Could you check a few things on this model? Use its own coordinates, in mm. Round coordinates to 2 decimals unless told otherwise and drop trailing zeros. Loops run counter-clockwise (first coordinate to the right, second up) from the corner with the lowest first, then second, coordinate; pieces in that order, holes last. Notation, with made-up numbers: M 50,17.5 L 70,17.5 A22 ccw 70,27.5 Z; hole C 82,-33 d4. An arc over 180 degrees is marked long. Return JSON: item names as keys, results as strings. Group by question number.
Autodesk Inventor part; units mm, degrees
ref_plane "Начальная плоскость" through (0, 0, -68.5714) normal (0, 0, 1) x (1, 0, 0)
ref_plane "Конечная плоскость" through (0, 0, 2801.8221) normal (0, 0, 1) x (1, 0, 0)
ref_plane "РабПлоскость4" through (91.07, -73.4212, 2735.6598) normal (0, -0.5039, 0.8638) x (1, 0, 0)
ref_plane "Начальная плоскость" through (0, 0, -68.5714) normal (0, 0, 1) x (1, 0, 0)
ref_plane "Конечная плоскость" through (0, 0, 2801.8221) normal (0, 0, 1) x (1, 0, 0)
sketch "Эскиз" plane through (0, 0, 0) normal (0, 0, 1) x (1, 0, 0)
  line L0 (-1.43, 0) -> (-1.43, 40)
  line L1 (-1.43, 40) -> (43.57, 40)
  line L2 (43.57, 40) -> (43.57, 38.1774)
  line L3 (39.9881, 34.1993) -> (11.2338, 31.1771)
  line L4 (4.07, 23.221) -> (4.07, 0)
  line L5 (4.07, 0) -> (-1.43, 0) construction
  line L6 (23.82, 40) -> (23.82, 32.5) construction
  line L7 (43.57, 34.5758) -> (43.57, 32.5) construction
  line L8 (43.57, 32.5) -> (23.82, 32.5) construction
  line L9 (0, 15) -> (0, -27) construction
  line L10 (-5.539, 0) -> (16.0067, 0) construction
  line L11 (-1.43, 0) -> (-1.43, -40)
  line L12 (-1.43, -40) -> (43.57, -40)
  line L13 (43.57, -40) -> (43.57, -38.1774)
  line L14 (39.9881, -34.1993) -> (11.2338, -31.1771)
  line L15 (4.07, -23.221) -> (4.07, 0)
  arc A0 (11.2338, 31.1771) -> (4.07, 23.221) centre (12.07, 23.221) ccw
  arc A1 (4.07, -23.221) -> (11.2338, -31.1771) centre (12.07, -23.221) ccw
  arc A2 (39.9881, 34.1993) -> (43.57, 38.1774) centre (39.57, 38.1774) ccw
  arc A3 (43.57, -38.1774) -> (39.9881, -34.1993) centre (39.57, -38.1774) ccw
  line L16 (0, 56) -> (0, -56) construction
  line L17 (-15.5135, 0) -> (54.308, 0) construction
  point P0 (4.07, 30.4242)
  point P1 (43.57, -34.5758)
  point P2 (4.07, -30.4242)
  point P3 (23.82, -40)
  point P4 (23.82, -32.5)
  dimension "d0" = 5.5
  dimension "d1" = 40
  dimension "d2" = 45
  dimension "d3" = 7.5
  dimension "d4" = 19.75
  dimension "d5" = 2.0758
  dimension "d23" = 8
  dimension "d24" = 4
  dimension "d25" = 1.43
extrude "Тело" add sketch "Эскиз" along normal up to surface (2870.3936 mm away) from surface at -68.5714
sketch "Sketch3" plane through (0, 0, 0) normal (0, 0, 1) x (1, 0, 0)
  line L0 (0, 0) -> (10, 0)
ref_plane "Work Plane3" through (0, 0, 0) normal (0, -1, 0) x (1, 0, 0)
sketch "Sketch4" plane through (0, 0, 0) normal (0, -1, 0) x (1, 0, 0)
  line L0 (-2, -68.5714) -> (12, -68.5714)
  line L1 (-2, 2801.8221) -> (12, 2801.8221)
  dimension "d29" = 2870.3936
ref_plane "РабПлоскость4" through (91.07, -73.4212, 2735.6598) normal (0, -0.5039, 0.8638) x (1, 0, 0)
split "Разделение1" plane through (91.07, -73.4212, 2735.6598) removes the side toward (0, -0.5039, 0.8638)
ref_plane "РабПлоскость5" through (91.07, -20.1548, 34.5512) normal (0, -0.8638, -0.5039) x (1, 0, 0)
split "Разделение2" plane through (91.07, -20.1548, 34.5512) removes the side toward (0, -0.8638, -0.5039)
equation "\"d0\" = G_T"
equation "\"d1\" = 0.5 * G_H"
equation "\"d2\" = G_W"
equation "\"d3\" = G_T1"
equation "\"d4\" = G_C"
equation "\"d23\" = G_IR"
equation "\"d24\" = G_ER"
equation "\"d25\" = ex"
equation "\"d6\" = G_L"
equation "\"G_W\" = 45"
equation "\"G_T\" = 5.5"
equation "\"G_T1\" = 7.5"
equation "\"G_NG\" = 0.105104"
equation "\"G_ER\" = 4"
equation "\"G_IR\" = 8"
equation "\"G_C\" = 19.75"
equation "\"G_L\" = d29"
equation "\"ex\" = 1.43"
equation "\"G_OFFSET_START\" = 68.57143"
equation "\"G_OFFSET_END\" = 23.33333"
equation "\"d26\" = -G_OFFSET_START"
equation "\"d27\" = G_OFFSET_END + B_L"
equation "\"B_L\" = 2778.4888"
properties part number "ISO 657/11 - CH 80 x 8 - 2870,39" material "Сталь, мягкая"
1. If we section it at B-B, the plane z = 1691.5: Please give me the cut outline in (x, y).
2. If we section it at C-C, the plane y = -2: Please give me the cut outline in (x, z).
3. We'd pull the mould along Y, two halves only. Please class faces 1 (the face through (21, 40, 1347)), 2 (the face through (-1.43, -1, 1347)), 3 (the face through (4.07, 0, 1356)): +Y half, -Y half, draft (parallel to the pull), parting line (faces both ways), or undercut.
4. I'm going to push flat-ended pins straight in: pin 1 Ø4 at (y, z) = (-9, 243.5) entering from +X; pin 2 Ø5 at (x, y) = (19.5, -31) entering from +Z. Where does each tip first touch, or does it pass through?
5. I need wall thicknesses on probe 1 along Y at (x, z) = (40, 956.5); probe 2 along Y at (x, z) = (40.5, 2465); probe 3 along X at (y, z) = (22.5, 907.5). Which ranges of each line are inside material? Lowest first, please.
Geometry results:
{
 "1": {"outline": "M -1.43,-40 L 43.57,-40 L 43.57,-38.18 A4 ccw 39.99,-34.2 L 11.23,-31.18 A8 cw 4.07,-23.22 L 4.07,23.22 A8 cw 11.23,31.18 L 39.99,34.2 A4 ccw 43.57,38.18 L 43.57,40 L -1.43,40 Z"},
 "2": {"outline": "M -1.43,3.43 L 4.07,3.43 L 4.07,2777.32 L -1.43,2777.32 Z"},
 "3": {"face 1": "+Y half", "face 2": "draft", "face 3": "undercut"},
 "4": {"pin 1": "x = 4.07", "pin 2": "z = 2759.94"},
 "5": {"probe 1": "-40 to -34.2, 34.2 to 40", "probe 2": "-40 to -34.29, 34.29 to 40", "probe 3": "-1.43 to 4.07"}
}
